CAD build for the part. Positions are in the model's coordinates, mm. Face numbers are marked on the shaded views. Give positions to 0.01 mm unless a question says otherwise; leave off trailing zeros. Write each loop counter-clockwise with the first axis right and the second up, starting at its lowest first coordinate (ties: lowest second). Pieces come first, ordered by that corner, then holes. Notation, with made-up numbers: (7, 49.25) -> (59, 49.25) arc R13 cw to (59, 64.25) -> close; hole circle Ø6 at (52.25, 10). An arc over 180 degrees is marked (long way). Answer as a JSON object with one key per item and string values.
```python
from build123d import *

# Parameters (mm, degrees)
EXTRUDE_1_DEPTH           = 805
EXTRUDE_2_DEPTH           = 805
EXTRUDE_3_DEPTH           = 805
CUT_EXTRUDE_1_DEPTH       = 892.299051946
CUT_EXTRUDE_1_DEPTH_BACK  = 892.299051946
SKETCH_4_W                = 121.26524617
SKETCH_4_H                = 160
CUT_EXTRUDE_2_DEPTH       = 892.299051946
CUT_EXTRUDE_2_DEPTH_BACK  = 892.299051946
SKETCH_5_R                = 80
CUT_EXTRUDE_3_DEPTH       = 892.299051946
CUT_EXTRUDE_3_DEPTH_BACK  = 892.299051946
SKETCH_6_R                = 95
CUT_EXTRUDE_4_DEPTH       = 892.299051946
CUT_EXTRUDE_4_DEPTH_BACK  = 892.299051946
SKETCH_7_R                = 15
CUT_EXTRUDE_5_DEPTH       = 892.299051946
CUT_EXTRUDE_5_DEPTH_BACK  = 892.299051946
SKETCH_8_R                = 5.25
CUT_EXTRUDE_6_DEPTH       = 892.299051946
CUT_EXTRUDE_6_DEPTH_BACK  = 892.299051946
SKETCH_9_R                = 8.75
CUT_EXTRUDE_7_DEPTH       = 892.299051946
CUT_EXTRUDE_7_DEPTH_BACK  = 892.299051946
SKETCH_10_R               = 10
CUT_EXTRUDE_8_DEPTH       = 892.299051946
CUT_EXTRUDE_8_DEPTH_BACK  = 892.299051946
SKETCH_11_R               = 7
CUT_EXTRUDE_9_DEPTH       = 892.299051946
CUT_EXTRUDE_9_DEPTH_BACK  = 892.299051946
SKETCH_12_R               = 3.4
CUT_EXTRUDE_10_DEPTH      = 892.299051946
CUT_EXTRUDE_10_DEPTH_BACK = 892.299051946
SKETCH_13_R               = 5.25
CUT_EXTRUDE_11_DEPTH      = 892.299051946
CUT_EXTRUDE_11_DEPTH_BACK = 892.299051946
SKETCH_14_R               = 2.5
CUT_EXTRUDE_12_DEPTH      = 892.299051946
CUT_EXTRUDE_12_DEPTH_BACK = 892.299051946
SKETCH_15_R               = 5.7225
CUT_EXTRUDE_13_DEPTH      = 892.299051946
CUT_EXTRUDE_13_DEPTH_BACK = 892.299051946
SKETCH_16_R               = 7
CUT_EXTRUDE_14_DEPTH      = 892.299051946
CUT_EXTRUDE_14_DEPTH_BACK = 892.299051946
SKETCH_17_R               = 7
SKETCH_19_R               = 2.5
CUT_EXTRUDE_16_DEPTH      = 15
SKETCH_20_R               = 2.5
CUT_EXTRUDE_17_DEPTH      = 55
CUT_EXTRUDE_START         = -15
SKETCH_21_R               = 2.5
CUT_EXTRUDE_18_DEPTH      = 15
SKETCH_23_R               = 2.5
CUT_EXTRUDE_20_DEPTH      = 15
SKETCH_25_R               = 2.5
CUT_EXTRUDE_22_DEPTH      = 68
SKETCH_27_R               = 2.1
CUT_EXTRUDE_24_DEPTH      = 71


with BuildPart() as part:
    # ｽｹｯﾁ1 → ﾎﾞｽ - 押し出し1 (new body)
    with BuildSketch(Plane(origin=(0, 0, 0), x_dir=(1, 0, 0), z_dir=(0, 1, 0))):
        Polygon((-336, 37), (-322.5, 37), (-322.5, 40), (322.5, 40), (322.5, 37), (336, 37), (336, 82), (305, 82), (305, 79), (-305, 79), (-305, 82), (-336, 82), align=None)
    extrude(amount=EXTRUDE_1_DEPTH)

    # ｽｹｯﾁ2 → ﾎﾞｽ - 押し出し2 (add)
    with BuildSketch(Plane(origin=(0, 0, 0), x_dir=(1, 0, 0), z_dir=(0, 1, 0))):
        Polygon((-355, 0), (-336, 0), (-336, 135), (-358, 135), (-358, 125), (-355, 125), align=None)
    extrude(amount=EXTRUDE_2_DEPTH)

    # ｽｹｯﾁ3 → ﾎﾞｽ - 押し出し3 (add)
    with BuildSketch(Plane(origin=(0, 0, 0), x_dir=(1, 0, 0), z_dir=(0, 1, 0))):
        Polygon((355, 0), (336, 0), (336, 135), (358, 135), (358, 125), (355, 125), align=None)
    extrude(amount=EXTRUDE_3_DEPTH)

    # ｽｹｯﾁ4 → ｶｯﾄ - 押し出し1 (cut, two sides: drawn at the far end of the back side and taken through both)
    with BuildSketch(Plane.XY.offset(-CUT_EXTRUDE_1_DEPTH_BACK)):
        with Locations((60.632623085, 400)):
            Rectangle(SKETCH_4_W, SKETCH_4_H)
    extrude(amount=CUT_EXTRUDE_1_DEPTH + CUT_EXTRUDE_1_DEPTH_BACK, mode=Mode.SUBTRACT)

    # ｽｹｯﾁ5 → ｶｯﾄ - 押し出し2 (cut, two sides: drawn at the far end of the back side and taken through both)
    with BuildSketch(Plane.XY.offset(-CUT_EXTRUDE_2_DEPTH_BACK)):
        with Locations((0, 400)):
            Circle(SKETCH_5_R)
    extrude(amount=CUT_EXTRUDE_2_DEPTH + CUT_EXTRUDE_2_DEPTH_BACK, mode=Mode.SUBTRACT)

    # ｽｹｯﾁ6 → ｶｯﾄ - 押し出し3 (cut, two sides: drawn at the far end of the back side and taken through both)
    with BuildSketch(Plane.XY.offset(-CUT_EXTRUDE_3_DEPTH_BACK)):
        with Locations((172.5, 400)):
            Circle(SKETCH_6_R)
    extrude(amount=CUT_EXTRUDE_3_DEPTH + CUT_EXTRUDE_3_DEPTH_BACK, mode=Mode.SUBTRACT)

    # ｽｹｯﾁ7 → ｶｯﾄ - 押し出し4 (cut, two sides: drawn at the far end of the back side and taken through both)
    with BuildSketch(Plane.XY.offset(-CUT_EXTRUDE_4_DEPTH_BACK)):
        with Locations((-260, 400)):
            Circle(SKETCH_7_R)
    extrude(amount=CUT_EXTRUDE_4_DEPTH + CUT_EXTRUDE_4_DEPTH_BACK, mode=Mode.SUBTRACT)

    # ｽｹｯﾁ8 → ｶｯﾄ - 押し出し5 (cut, two sides: drawn at the far end of the back side and taken through both)
    with BuildSketch(Plane.XY.offset(-CUT_EXTRUDE_5_DEPTH_BACK)):
        with Locations((290.746961997, 500.112207496)):
            Circle(SKETCH_8_R)
        with Locations((230.303884143, 603.755664826)):
            Circle(SKETCH_8_R)
        with Locations((134.799127638, 676.379169237)):
            Circle(SKETCH_8_R)
        with Locations((18.772425907, 706.926450515)):
            Circle(SKETCH_8_R)
        with Locations((-100.112207496, 690.746961997)):
            Circle(SKETCH_8_R)
        with Locations((-203.755664826, 630.303884143)):
            Circle(SKETCH_8_R)
        with Locations((-276.379169237, 534.799127638)):
            Circle(SKETCH_8_R)
        with Locations((-290.746961997, 299.887792504)):
            Circle(SKETCH_8_R)
        with Locations((-230.303884143, 196.244335174)):
            Circle(SKETCH_8_R)
        with Locations((-134.799127638, 123.620830763)):
            Circle(SKETCH_8_R)
        with Locations((-18.772425907, 93.073549485)):
            Circle(SKETCH_8_R)
        with Locations((100.112207496, 109.253038003)):
            Circle(SKETCH_8_R)
        with Locations((203.755664826, 169.696115857)):
            Circle(SKETCH_8_R)
        with Locations((276.379169237, 265.200872362)):
            Circle(SKETCH_8_R)
    extrude(amount=CUT_EXTRUDE_5_DEPTH + CUT_EXTRUDE_5_DEPTH_BACK, mode=Mode.SUBTRACT)

    # ｽｹｯﾁ9 → ｶｯﾄ - 押し出し6 (cut, two sides: drawn at the far end of the back side and taken through both)
    with BuildSketch(Plane.XY.offset(-CUT_EXTRUDE_6_DEPTH_BACK)):
        with Locations((-205, 660)):
            Circle(SKETCH_9_R)
        with Locations((-205, 750)):
            Circle(SKETCH_9_R)
        with Locations((-35, 660)):
            Circle(SKETCH_9_R)
        with Locations((-35, 750)):
            Circle(SKETCH_9_R)
    extrude(amount=CUT_EXTRUDE_6_DEPTH + CUT_EXTRUDE_6_DEPTH_BACK, mode=Mode.SUBTRACT)

    # ｽｹｯﾁ10 → ｶｯﾄ - 押し出し7 (cut, two sides: drawn at the far end of the back side and taken through both)
    with BuildSketch(Plane.XY.offset(-CUT_EXTRUDE_7_DEPTH_BACK)):
        with Locations((-205, 705)):
            Circle(SKETCH_10_R)
        with Locations((-35, 705)):
            Circle(SKETCH_10_R)
    extrude(amount=CUT_EXTRUDE_7_DEPTH + CUT_EXTRUDE_7_DEPTH_BACK, mode=Mode.SUBTRACT)

    # ｽｹｯﾁ11 → ｶｯﾄ - 押し出し8 (cut, two sides: drawn at the far end of the back side and taken through both)
    with BuildSketch(Plane.XY.offset(-CUT_EXTRUDE_8_DEPTH_BACK)):
        with Locations((82.5, 285)):
            Circle(SKETCH_11_R)
        with Locations((262.5, 285)):
            Circle(SKETCH_11_R)
        with Locations((82.5, 515)):
            Circle(SKETCH_11_R)
        with Locations((262.5, 515)):
            Circle(SKETCH_11_R)
    extrude(amount=CUT_EXTRUDE_8_DEPTH + CUT_EXTRUDE_8_DEPTH_BACK, mode=Mode.SUBTRACT)

    # ｽｹｯﾁ12 → ｶｯﾄ - 押し出し9 (cut, two sides: drawn at the far end of the back side and taken through both)
    with BuildSketch(Plane.XY.offset(-CUT_EXTRUDE_9_DEPTH_BACK)):
        with Locations((82.5, 212.5)):
            Circle(SKETCH_12_R)
        with Locations((82.5, 247.5)):
            Circle(SKETCH_12_R)
        with Locations((82.5, 552.5)):
            Circle(SKETCH_12_R)
        with Locations((82.5, 587.5)):
            Circle(SKETCH_12_R)
    extrude(amount=CUT_EXTRUDE_9_DEPTH + CUT_EXTRUDE_9_DEPTH_BACK, mode=Mode.SUBTRACT)

    # ｽｹｯﾁ13 → ｶｯﾄ - 押し出し10 (cut, two sides: drawn at the far end of the back side and taken through both)
    with BuildSketch(Plane.XY.offset(-CUT_EXTRUDE_10_DEPTH_BACK)):
        with Locations((-40, 135)):
            Circle(SKETCH_13_R)
        with Locations((40, 135)):
            Circle(SKETCH_13_R)
    extrude(amount=CUT_EXTRUDE_10_DEPTH + CUT_EXTRUDE_10_DEPTH_BACK, mode=Mode.SUBTRACT)

    # ｽｹｯﾁ14 → ｶｯﾄ - 押し出し11 (cut, two sides: drawn at the far end of the back side and taken through both)
    with BuildSketch(Plane.XY.offset(-CUT_EXTRUDE_11_DEPTH_BACK)):
        with Locations((25, 640)):
            Circle(SKETCH_14_R)
        with Locations((25, 670)):
            Circle(SKETCH_14_R)
    extrude(amount=CUT_EXTRUDE_11_DEPTH + CUT_EXTRUDE_11_DEPTH_BACK, mode=Mode.SUBTRACT)

    # ｽｹｯﾁ15 → ｶｯﾄ - 押し出し12 (cut, two sides: drawn at the far end of the back side and taken through both)
    with BuildSketch(Plane.XY.offset(-CUT_EXTRUDE_12_DEPTH_BACK)):
        with Locations((48, 548)):
            Circle(SKETCH_15_R)
    extrude(amount=CUT_EXTRUDE_12_DEPTH + CUT_EXTRUDE_12_DEPTH_BACK, mode=Mode.SUBTRACT)

    # ｽｹｯﾁ16 → ｶｯﾄ - 押し出し13 (cut, two sides: drawn at the far end of the back side and taken through both)
    with BuildSketch(Plane.XY.offset(-CUT_EXTRUDE_13_DEPTH_BACK)):
        with Locations((-230, 785)):
            Circle(SKETCH_16_R)
        with Locations((230, 785)):
            Circle(SKETCH_16_R)
    extrude(amount=CUT_EXTRUDE_13_DEPTH + CUT_EXTRUDE_13_DEPTH_BACK, mode=Mode.SUBTRACT)

    # ｽｹｯﾁ17 → ｶｯﾄ - 押し出し14 (cut, two sides: drawn at the far end of the back side and taken through both)
    with BuildSketch(Plane(origin=(0, 0, 0), x_dir=(0, 0, -1), z_dir=(1, 0, 0)).offset(-CUT_EXTRUDE_14_DEPTH_BACK)):
        with Locations((15, 55)):
            Circle(SKETCH_17_R)
        with Locations((15, 135)):
            Circle(SKETCH_17_R)
        with Locations((15, 670)):
            Circle(SKETCH_17_R)
        with Locations((15, 750)):
            Circle(SKETCH_17_R)
        with Locations((115, 55)):
            Circle(SKETCH_17_R)
        with Locations((115, 135)):
            Circle(SKETCH_17_R)
        with Locations((115, 670)):
            Circle(SKETCH_17_R)
        with Locations((115, 750)):
            Circle(SKETCH_17_R)
    extrude(amount=CUT_EXTRUDE_14_DEPTH + CUT_EXTRUDE_14_DEPTH_BACK, mode=Mode.SUBTRACT)

    # ｽｹｯﾁ19 → ｶｯﾄ - 押し出し16 (cut)
    with BuildSketch(Plane(origin=(0, 0, 0), x_dir=(1, 0, 0), z_dir=(0, 1, 0))):
        with Locations(Location((-270, 48, 0), (0, 0, 270))):
            Circle(SKETCH_19_R)
        with Locations(Location((0, 48, 0), (0, 0, 270))):
            Circle(SKETCH_19_R)
        with Locations(Location((270, 48, 0), (0, 0, 270))):
            Circle(SKETCH_19_R)
    extrude(amount=CUT_EXTRUDE_16_DEPTH, mode=Mode.SUBTRACT)

    # ｽｹｯﾁ20 → ｶｯﾄ - 押し出し17 (cut)
    with BuildSketch(Plane.XY):
        with Locations((-280, 725)):
            Circle(SKETCH_20_R)
        with Locations((-280, 745)):
            Circle(SKETCH_20_R)
        with Locations((-280, 785)):
            Circle(SKETCH_20_R)
        with Locations((-250, 785)):
            Circle(SKETCH_20_R)
    extrude(amount=-CUT_EXTRUDE_17_DEPTH, mode=Mode.SUBTRACT)

    # ｽｹｯﾁ21 → ｶｯﾄ - 押し出し18 (cut)
    with BuildSketch(Plane(origin=(0, 805, 0), x_dir=(1, 0, 0), z_dir=(0, 1, 0)).offset(CUT_EXTRUDE_START)):
        with Locations(Location((-270, 48, 0), (0, 0, 270))):
            Circle(SKETCH_21_R)
        with Locations(Location((0, 48, 0), (0, 0, 270))):
            Circle(SKETCH_21_R)
        with Locations(Location((270, 48, 0), (0, 0, 270))):
            Circle(SKETCH_21_R)
    extrude(amount=CUT_EXTRUDE_18_DEPTH, mode=Mode.SUBTRACT)

    # ｽｹｯﾁ23 → ｶｯﾄ - 押し出し20 (cut)
    with BuildSketch(Plane.XY.offset(-135)):
        with Locations((-348, 38)):
            Circle(SKETCH_23_R)
        with Locations((-348, 158)):
            Circle(SKETCH_23_R)
    extrude(amount=CUT_EXTRUDE_20_DEPTH, mode=Mode.SUBTRACT)

    # ｽｹｯﾁ25 → ｶｯﾄ - 押し出し22 (cut)
    with BuildSketch(Plane.XY.offset(-135)):
        with Locations((-260, 370)):
            Circle(SKETCH_25_R)
        with Locations((-260, 430)):
            Circle(SKETCH_25_R)
    extrude(amount=CUT_EXTRUDE_22_DEPTH, mode=Mode.SUBTRACT)

    # ｽｹｯﾁ27 → ｶｯﾄ - 押し出し24 (cut)
    with BuildSketch(Plane.XY.offset(-135)):
        with Locations((135, 640)):
            Circle(SKETCH_27_R)
        with Locations((250, 640)):
            Circle(SKETCH_27_R)
    extrude(amount=CUT_EXTRUDE_24_DEPTH, mode=Mode.SUBTRACT)


solid = part.part
```
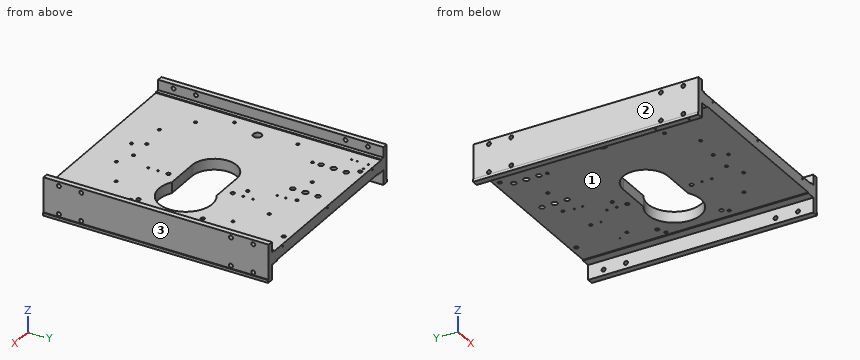
1) Wall check: probe 1 along X at (y, z) = (136, -51); probe 2 along Y at (x, z) = (343, -115); probe 3 along Z at (x, y) = (-341, 670). Give the ranges that are in metal, low to high.
Model answer:
{"probe 1": "x = -355 to -45.15, -34.85 to 34.85, 45.15 to 355", "probe 2": "y = 0 to 48, 62 to 128, 142 to 663, 677 to 743, 757 to 805", "probe 3": "z = -135 to -122, -108 to -22, -8 to 0"}
2) Slice it at A-A (z = -94). List the corners of the cut face in (x, y).
Model answer:
{"outline": "(-355, 0) -> (-336, 0) -> (-336, 805) -> (-355, 805) -> close; (336, 0) -> (355, 0) -> (355, 805) -> (336, 805) -> close"}
3) Mould opens along X. For the marked faces 1, 2 and 3 say: released by +X, released by -X, zero draft, split by the parting line, or undercut.
Model answer:
{"face 1": "undercut", "face 2": "released by -X", "face 3": "released by +X"}
4) Pin check, flat tips, straight feed: pin 1 (8 mm diameter, centred on x = -260, y = 370, fed in from +Z); pin 2 (2 mm diameter, centred on x = -199.5, y = 648.5, fed in from -Z); pin 3 (6 mm diameter, centred on x = -348, y = 158, fed in from -Z); pin 4 (2.5 mm diameter, centred on x = -280.5, y = 724, fed in from +Z). Stop position of each tip, or through.
Model answer:
{"pin 1": "stops at z = -40", "pin 2": "stops at z = -79", "pin 3": "stops at z = -135", "pin 4": "stops at z = -55"}
